Can you work these out from the model? Positions are in its coordinate system, mm. Face numbers are marked on the shaded views. A direction names the side the tool comes from. Give positions to 0.01 mm unless a question says otherwise; leave off trailing zeros. Order: outer loops, then holes, each group sorted by start corner. A loop starts at its lowest first (then second) coordinate and runs counter-clockwise, first axis right, second up. Notation, with made-up numbers: M -19.75,73 L -11.75,73 A29 cw -11.75,99 Z; hole C 36.5,-29 d11. An arc over 180 degrees is marked long. Use one line per item in the form item = value. Start each with the question number.
1. For the marked faces 1 and 2, which set-ups out of +Z, -Z, +X, -X, +Y, -Y let a thin tool reach every point of the face, with its end or its side?
2. I need wall thicknesses on L1, parallel to X at y = 39, z = 4.25; L2, parallel to Y at x = -24.95, z = 0; L3, parallel to Y at x = -25.55, z = 0. Which ranges of each line are inside material? Lowest first, please.
3. I want a section at D-D, the plane x = -15. List the corners of the cut face in (y, z) for me.
4. I want a section at C-C, the plane y = 44. List the corners of the cut face in (x, z) for me, and give its area (3 significant figures).
5. I want a section at B-B, the plane y = 13. List the corners of the cut face in (x, z) for me, and give its area (3 significant figures).
6. Will these pins go through, and if not, where does the flat tip stop? P1, Ø1.9, axis at y = 54.39, z = 0, coming from the -X side; P2, Ø3, axis at x = 0.5, z = -9, coming from the +Y side; P3, Ø10.5, axis at y = 46.06, z = 0, coming from the +X side; P4, Ø12, axis at x = 19.5, z = 6, coming from the +Y side.
7. I want a section at A-A, the plane x = 0. List the corners of the cut face in (y, z) for me (1 decimal), and give its area (3 significant figures).
8. We'd pull the mould along X, two halves only. Please class the marked faces 3, 4, 5 and 6: +X half, -X half, draft (parallel to the pull), parting line (faces both ways), or undercut.
```python
from build123d import *

# Parameters (mm, degrees)
SKETCH1_W               = 49.1998
SKETCH1_H               = 24.6126
SKETCH1_R               = 1.1938
SKETCH1_R_2             = 4.0005
EXTRUDE1_DEPTH          = 1.524
SKETCH1_3_W             = 1.524
SKETCH1_3_H             = 24.6126
EXTRUDE2_DEPTH          = 58.3438
SKETCH4_R               = 4.0005
SKETCH4_R_2             = 1.1938
CUT_EXTRUDE1_DEPTH      = 40.8686
CUT_EXTRUDE1_DEPTH_BACK = 40.8686
FILLET1_R               = 0.254
FILLET2_R               = 1.778


with BuildPart() as part:
    # Sketch1 → Extrude1 (new body)
    with BuildSketch(Plane(origin=(0, 0, 0), x_dir=(1, 0, 0), z_dir=(0, 1, 0))):
        Rectangle(SKETCH1_W, SKETCH1_H)
        with Locations((-8.3312, 0)):
            Circle(SKETCH1_R, mode=Mode.SUBTRACT)
        with Locations((0, -8.3312)):
            Circle(SKETCH1_R, mode=Mode.SUBTRACT)
        Circle(SKETCH1_R_2, mode=Mode.SUBTRACT)
        with Locations((8.3312, 0)):
            Circle(SKETCH1_R, mode=Mode.SUBTRACT)
        with Locations((0, 8.3312)):
            Circle(SKETCH1_R, mode=Mode.SUBTRACT)
    extrude(amount=EXTRUDE1_DEPTH)

    # Sketch1<3> → Extrude2 (add)
    with BuildSketch(Plane(origin=(0, 0, 0), x_dir=(1, 0, 0), z_dir=(0, 1, 0))):
        with Locations((25.3619, 0)):
            Rectangle(SKETCH1_3_W, SKETCH1_3_H)
        with Locations((-25.3619, 0)):
            Rectangle(SKETCH1_3_W, SKETCH1_3_H)
    extrude(amount=EXTRUDE2_DEPTH)

    # Sketch4 → Cut-Extrude1 (cut, two sides)
    with BuildSketch(Plane(origin=(0, 0, 0), x_dir=(0, 0, -1), z_dir=(1, 0, 0))) as cut_extrude1_sk:
        with BuildLine():
            Line((-0.5589443, 58.3438), (-12.3063, 58.3438))
            Line((-12.3063, 58.3438), (-12.3063, 46.0502))
            ThreePointArc((-12.3063, 46.0502), (-8.897290484, 54.552155171), (-0.5589443, 58.3438))
        make_face()
        with BuildLine():
            Line((12.3063, 58.3438), (0.5589443, 58.3438))
            ThreePointArc((0.5589443, 58.3438), (8.897290484, 54.552155171), (12.3063, 46.0502))
            Line((12.3063, 46.0502), (12.3063, 58.3438))
        make_face()
        with Locations((0, 46.0629)):
            Circle(SKETCH4_R)
        with Locations((8.3312, 46.0629)):
            Circle(SKETCH4_R_2)
        with Locations((0, 54.3941)):
            Circle(SKETCH4_R_2)
        with Locations((-8.3312, 46.0629)):
            Circle(SKETCH4_R_2)
        with Locations((0, 37.7317)):
            Circle(SKETCH4_R_2)
    extrude(amount=CUT_EXTRUDE1_DEPTH, mode=Mode.SUBTRACT)
    extrude(cut_extrude1_sk.sketch, amount=-CUT_EXTRUDE1_DEPTH_BACK, mode=Mode.SUBTRACT)

    # Fillet1
    fillet1_edges = [part.edges().sort_by_distance(p)[0] for p in [
        (-24.5999, 1.524, 0),
        (24.5999, 1.524, 0),
    ]]
    fillet(fillet1_edges, radius=FILLET1_R)

    # Fillet2
    fillet2_edges = [part.edges().sort_by_distance(p)[0] for p in [
        (-26.1239, 0, 0),
        (26.1239, 0, 0),
    ]]
    fillet(fillet2_edges, radius=FILLET2_R)


solid = part.part
```
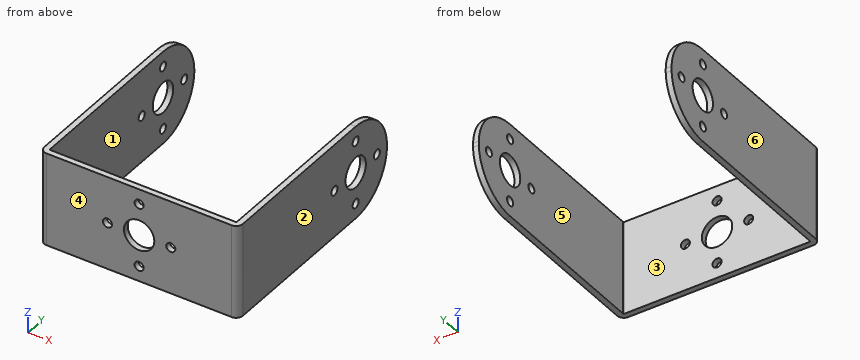
Check result:
q1.face_1 = +Z, -Z, +Y
q1.face_2 = +Z, -Z, +X, +Y, -Y
q2.L1 = -26.12 to -24.6, 24.6 to 26.12
q2.L2 = 0.11 to 36.54, 38.93 to 42.06, 50.06 to 53.2, 55.59 to 58.34
q2.L3 = 0.47 to 36.54, 38.93 to 42.06, 50.06 to 53.2, 55.59 to 58.34
q3.outline = M 0,-12.31 L 1.52,-12.31 L 1.52,12.31 L 0,12.31 Z
q4.outline = M -26.12,-12.31 L -24.6,-12.31 L -24.6,-3.43 L -26.12,-3.43 Z; M -26.12,3.43 L -24.6,3.43 L -24.6,12.31 L -26.12,12.31 Z; M 24.6,-12.31 L 26.12,-12.31 L 26.12,-3.43 L 24.6,-3.43 Z; M 24.6,3.43 L 26.12,3.43 L 26.12,12.31 L 24.6,12.31 Z
q4.area = 54.1 mm2
q5.outline = M -26.12,-12.31 L -24.6,-12.31 L -24.6,12.31 L -26.12,12.31 Z; M 24.6,-12.31 L 26.12,-12.31 L 26.12,12.31 L 24.6,12.31 Z
q5.area = 75.0 mm2
q6.P1 = through
q6.P2 = 1.52
q6.P3 = 26.12
q6.P4 = 58.02
q7.outline = M 0,-12.3 L 1.5,-12.3 L 1.5,-9.5 L 0,-9.5 Z; M 0,-7.1 L 1.5,-7.1 L 1.5,-4 L 0,-4 Z; M 0,4 L 1.5,4 L 1.5,7.1 L 0,7.1 Z; M 0,9.5 L 1.5,9.5 L 1.5,12.3 L 0,12.3 Z
q7.area = 18.0 mm2
q8.face_3 = undercut
q8.face_4 = draft
q8.face_5 = undercut
q8.face_6 = -X half
